Autodesk Fusion 360 part; units mm, degrees
sketch "Sketch1" plane through (0, 0, 0) normal (0, 0, 1) x (1, 0, 0)
  line L0 (0, 0) -> (203, 0) construction
  line L1 (203, 0) -> (203, 151) construction
  line L2 (203, 151) -> (0, 151) construction
  line L3 (0, 151) -> (0, 0) construction
  line L4 (101.5, 151) -> (101.5, 0) construction
  line L5 (0, 75.5) -> (203, 75.5) construction
  circle A0 centre (25.85, 110.5) radius 2
  circle A1 centre (61.05, 125.25) radius 2
  circle A2 centre (21, 75.5) radius 2
  circle A3 centre (101.5, 125.25) radius 2
  circle A4 centre (141.95, 125.25) radius 2
  circle A5 centre (177.15, 110.5) radius 2
  circle A6 centre (182, 75.5) radius 2
  circle A7 centre (25.85, 40.5) radius 2
  circle A8 centre (101.5, 25.75) radius 2
  circle A9 centre (61.05, 25.75) radius 2
  circle A10 centre (141.95, 25.75) radius 2
  circle A11 centre (177.15, 40.5) radius 2
  line L6 (122.4543, 101.192) -> (171.4543, 101.192) construction
  line L7 (171.4543, 101.192) -> (171.4543, 43.192) construction
  line L8 (171.4543, 43.192) -> (122.4543, 43.192) construction
  line L9 (122.4543, 43.192) -> (122.4543, 101.192) construction
  line L10 (118.9543, 124.692) -> (174.9543, 124.692) construction
  line L11 (174.9543, 124.692) -> (174.9543, 39.692) construction
  line L12 (174.9543, 39.692) -> (118.9543, 39.692) construction
  line L13 (118.9543, 39.692) -> (118.9543, 124.692) construction
  circle A12 centre (122.4543, 101.192) radius 1.15
  circle A13 centre (171.4543, 101.192) radius 1.15
  circle A14 centre (171.4543, 43.192) radius 1.15
  circle A15 centre (122.4543, 43.192) radius 1.15
  circle A16 centre (122.4543, 101.192) radius 2.65
  circle A17 centre (171.4543, 101.192) radius 2.65
  circle A18 centre (171.4543, 43.192) radius 2.65
  circle A19 centre (122.4543, 43.192) radius 2.65
  line L14 (55.9879, 132.0749) -> (188.973, 132.0749)
  line L15 (188.973, 132.0749) -> (188.973, 17.4198)
  line L16 (188.973, 17.4198) -> (55.9879, 17.4198)
  line L17 (55.9879, 17.4198) -> (55.9879, 132.0749)
  line L18 (69.6743, 109.192) -> (87.4543, 109.192) construction
  line L19 (87.4543, 109.192) -> (87.4543, 63.472) construction
  line L20 (87.4543, 63.472) -> (69.6743, 63.472) construction
  line L21 (69.6743, 63.472) -> (69.6743, 109.192) construction
  circle A20 centre (69.6743, 109.192) radius 1.15
  circle A21 centre (69.6743, 109.192) radius 2.65
  circle A22 centre (87.4543, 109.192) radius 2.65
  circle A23 centre (87.4543, 109.192) radius 1.15
  circle A24 centre (69.6743, 63.472) radius 2.65
  circle A25 centre (69.6743, 63.472) radius 1.15
  circle A26 centre (87.4543, 63.472) radius 2.65
  circle A27 centre (87.4543, 63.472) radius 1.15
  line L22 (95.4972, 94.9899) -> (175.7715, 94.9899)
  line L23 (175.7715, 94.9899) -> (175.7715, 49.2006)
  line L24 (175.7715, 49.2006) -> (95.4972, 49.2006)
  line L25 (95.4972, 49.2006) -> (95.4972, 94.9899)
  point P0 (61.05, 125.25)
  point P1 (25.85, 110.5)
  point P2 (177.15, 110.5)
  point P3 (141.95, 125.25)
  point P4 (177.15, 40.5)
  point P5 (141.95, 25.75)
  point P6 (61.05, 25.75)
  point P7 (25.85, 40.5)
  point P8 (101.5, 125.25)
  point P9 (21, 75.5)
  point P10 (182, 75.5)
  point P11 (101.5, 25.75)
  point P12 (61.05, 25.75)
  point P13 (141.95, 25.75)
  point P14 (177.15, 40.5)
  dimension "d1" = 203
  dimension "d2" = 151
  dimension "d3" = 161
  dimension "d4" = 151.3
  dimension "d5" = 80.9
  dimension "d6" = 70
  dimension "d7" = 99.5
  dimension "d8" = 99.5
  dimension "d10" = 4
  dimension "d12" = 4
  dimension "d14" = 4
  dimension "d16" = 4
  dimension "d19" = 49
  dimension "d20" = 58
  dimension "d21" = 56
  dimension "d22" = 85
  dimension "d23" = 3.5
  dimension "d24" = 3.5
  dimension "d25" = 2.3
  dimension "d26" = 2.3
  dimension "d27" = 2.3
  dimension "d28" = 2.3
  dimension "d29" = 1.5
  dimension "d30" = 1.5
  dimension "d31" = 1.5
  dimension "d32" = 1.5
  dimension "d41" = 45.72
  dimension "d42" = 17.78
  dimension "d43" = 2.3
  dimension "d44" = 1.5
  dimension "d47" = 17.78
  dimension "d48" = -45.72
  dimension "d54" = 35
  dimension "d55" = 8
extrude "Extrude2" add sketch "Sketch1" along normal blind 1.5 contours A1 | A4 | A5 | A9 | A10 | A11 | A16 | A17 | A18 | A19 | L14 L15 L16 L17 | A21 | A22 | A24 | A25 | A26
extrude "Extrude3" add sketch "Sketch1" along normal blind 6 contours A16 | A17 | A18 | A19 | A21 | A22 | A26
draft "Draft1" angle 30 neutral plane through (0, 0, 6) pull (0, 0, 1) 7 faces at (120.1931, 102.5738, 3) (171.5204, 103.8412, 3) (171.5204, 45.8412, 3) (125.0912, 43.4559, 3) (71.9356, 110.5738, 3) (89.7156, 110.5738, 3) (90.0912, 63.7359, 3)
fillet "Fillet1" radius 10 8 edges at (55.9879, 17.4198, 0.75) (188.973, 17.4198, 0.75) (188.973, 132.0749, 0.75) (55.9879, 132.0749, 0.75) (95.4972, 94.9899, 0.75) (95.4972, 49.2006, 0.75) (175.7715, 94.9899, 0.75) (175.7715, 49.2006, 0.75)
Could you check a few things on this model? Use its own coordinates, in mm. A direction names the side the tool comes from. Give positions to 0.01 mm unless a question says otherwise; leave off trailing zeros. Write each loop counter-clockwise with the first axis right and the second up, starting at its lowest first coordinate (ties: lowest second). Pieces come first, ordered by that corner, then holes. Notation, with made-up numbers: (-23, -8) -> (-3, -8) arc R26 cw to (-3, 6) -> close; hole circle Ø3 at (-38.75, 65). An arc over 180 degrees is marked (long way). Answer as a JSON object with one key per item and string values.
Q1. Suppose I cut it at D-D on x = 101.5. Write out the boundary of the cut face in (y, z), then the cut area to 3 significant figures.
Taken from the geometry:
{"outline": "(17.42, 0) -> (23.75, 0) -> (23.75, 1.5) -> (17.42, 1.5) -> close; (27.75, 0) -> (50.03, 0) -> (50.03, 1.5) -> (27.75, 1.5) -> close; (94.16, 0) -> (123.25, 0) -> (123.25, 1.5) -> (94.16, 1.5) -> close; (127.25, 0) -> (132.07, 0) -> (132.07, 1.5) -> (127.25, 1.5) -> close", "area": "93.8 mm²"}
Q2. Which directions (+Z, -Z, +X, -X, +Y, -Y) give clear straight access to the entire face, cutting with the end or side of a thin tool? Please do faces 1 (the cylindrical face through (98.504, 92.138, 0.76)), 2 (the flat face through (173, 101, 6)), 3 (the flat face through (92, 76, 1.5)).
Taken from the geometry:
{"face 1": "+Z, -Z", "face 2": "+Z, +X, -X, +Y, -Y", "face 3": "+Z"}
Q3. Suppose I cut it at A-A on z = 2.4. Count the separate pieces of the cut face and the enclosed holes in it, then the cut area to 3 significant figures.
Taken from the geometry:
{"separate pieces": "7", "enclosed holes": "7", "area": "463 mm²"}
Q4. Will these pins go through, and if not, where does the flat tip stop? pin 1 Ø1.8 at (x, y) = (87.45, 63.47) entering from +Z; pin 2 Ø5 at (x, y) = (182, 75.5) entering from +Z.
Taken from the geometry:
{"pin 1": "passes through", "pin 2": "stops at z = 1.5"}
Q5. Suppose I cut it at C-C on x = 130. Write out the boundary of the cut face in (y, z).
Taken from the geometry:
{"outline": "(17.42, 0) -> (49.2, 0) -> (49.2, 1.5) -> (17.42, 1.5) -> close; (94.99, 0) -> (132.07, 0) -> (132.07, 1.5) -> (94.99, 1.5) -> close"}
Q6. Suppose I cut it at B-B on y = 75.5. Write out the boundary of the cut face in (x, z), then the cut area to 3 significant figures.
Taken from the geometry:
{"outline": "(55.99, 0) -> (95.5, 0) -> (95.5, 1.5) -> (55.99, 1.5) -> close; (175.77, 0) -> (180, 0) -> (180, 1.5) -> (175.77, 1.5) -> close; (184, 0) -> (188.97, 0) -> (188.97, 1.5) -> (184, 1.5) -> close", "area": "73.1 mm²"}
Q7. We'd pull the mould along X, two halves only. Please class faces 4 (the flat face through (123, 100, 6)), 5 (the cylindrical face through (185.966, 20.271, 0.76)), 6 (the conical face through (87.1, 106.1, 5.2)): released by +X, released by -X, zero draft, split by the parting line, or undercut.
Taken from the geometry:
{"face 4": "zero draft", "face 5": "released by +X", "face 6": "undercut"}
Q8. Please list where these lines run through material, in increasing order: L1, parallel to X at y = 101.5, z = 3.95; L2, parallel to X at y = 105, z = 2.35 (3 decimals); L3, parallel to X at y = 108.5, z = 0.65.
Taken from the geometry:
{"L1": "x = 118.63 to 121.35, 123.56 to 126.28, 167.63 to 170.35, 172.56 to 175.28", "L2": "x = 67.425 to 71.924, 85.205 to 89.704, 119.603 to 125.306, 168.603 to 174.306", "L3": "x = 55.99 to 68.76, 70.59 to 86.54, 88.37 to 188.97"}
